Input: part model. Units: mm. Frame: model coordinates. A direction names the side the tool comes from. Coordinates: 2 decimals unless noted, no trailing zeros. Write each loop counter-clockwise with the first axis right and the second up, starting at its lowest first coordinate (ties: lowest second). Pieces come first, ordered by that corner, then holes. Notation, with made-up numbers: M 23.5,23.5 L 37.5,23.5 A22 cw 37.5,32.5 Z; hole C -40,51.25 d1. An arc over 180 degrees is marked long. Write each question's results on one line, items separated by ' | '. Start each with the question number.
1. Set-up query: faces 3 (the flat face through (28, 9.5, 3)), 4 (the flat face through (-8, 20, -2.5)), 5 (the flat face through (-0.899, 32.177, 10.325)). Return all of +Z, -Z, +X, -X, +Y, -Y with unobstructed straight access to the full face (end or side cutting, diameter ignored); none if empty.
2. Ray query, probe 1 along Z at (x, y) = (0.5, 2.8); probe 2 along X at (y, z) = (10, -4); probe 3 along X at (y, z) = (8, -1). Return the intervals inside material, ascending.
3. Section query A-A, the plane x = 0.5. Count the separate pieces of the cut face and the enclosed holes in it, and give its area (3 significant figures).
4. Section query D-D, the plane y = 8.5. Output: boundary loops of the cut face in (x, z), and give its area (3 significant figures).
5. Pull-direction query (X, two-part tool) for faces 1 (the flat face through (12.79, 11.83, -0.26)), 2 (the flat face through (28, 7.5, 3)); classes: +X half, -X half, draft (parallel to the pull), parting line (faces both ways), or undercut.
6. Section query B-B, the plane z = 3.5. Output: boundary loops of the cut face in (x, y), and give its area (3 significant figures).
7. First-contact query: pin 1 (1.5 mm diameter, centred on x = -12.5, y = 33, fed in from +Z); pin 2 (12 mm diameter, centred on x = -17, z = -11.5, fed in from +Y); pin 3 (2.5 mm diameter, centred on x = 24, y = 8, fed in from -Z). Flat tips, straight axial feed; report the tip coordinate or a pass-through.
```python
from build123d import *

# Parameters (mm, degrees)
SKETCH2_W           = 58
SKETCH2_H           = 37
BOSS_EXTRUDE1_DEPTH = 17
BOSS_EXTRUDE2_DEPTH = 58
SKETCH4_R           = 12.5
BOSS_EXTRUDE3_DEPTH = 17
CUT_EXTRUDE1_DEPTH  = 38
SKETCH6_R           = 4.076
CUT_EXTRUDE2_DEPTH  = 23
SKETCH7_R           = 7.5075
SKETCH7_R_2         = 5.15
CUT_EXTRUDE3_DEPTH  = 59
SKETCH8_R           = 1.875
CUT_EXTRUDE4_DEPTH  = 59
SKETCH12_W          = 2
SKETCH12_H          = 2
CUT_EXTRUDE6_DEPTH  = 8
CUT_EXTRUDE7_DEPTH  = 57
SKETCH14_R          = 1.5
CUT_EXTRUDE8_DEPTH  = 35.5


with BuildPart() as part:
    # Sketch2 → Boss-Extrude1 (new body)
    with BuildSketch(Plane(origin=(0, 0, 0), x_dir=(1, 0, 0), z_dir=(0, 1, 0))):
        Rectangle(SKETCH2_W, SKETCH2_H)
    extrude(amount=BOSS_EXTRUDE1_DEPTH)

    # Sketch3 → Boss-Extrude2 (add)
    with BuildSketch(Plane(origin=(29, 0, 0), x_dir=(0, 0, -1), z_dir=(1, 0, 0))):
        with BuildLine():
            Line((-18.5, 23.5), (-18.5, 17))
            Line((-18.5, 17), (2.5, 17))
            Line((2.5, 17), (2.5, 23.5))
            ThreePointArc((2.5, 23.5), (-8, 34), (-18.5, 23.5))
        make_face()
    extrude(amount=-BOSS_EXTRUDE2_DEPTH)

    # Sketch4 → Boss-Extrude3 (add)
    with BuildSketch(Plane(origin=(29, 0, 0), x_dir=(0, 0, -1), z_dir=(1, 0, 0))):
        with Locations((7.043560763, 22)):
            Circle(SKETCH4_R)
    extrude(amount=-BOSS_EXTRUDE3_DEPTH)

    # Sketch5 → Cut-Extrude1 (cut, through all)
    with BuildSketch(Plane(origin=(0, 0, -18.5), x_dir=(-1, 0, 0), z_dir=(0, 0, -1))):
        Polygon((-15.5, 6.5), (-15.5, 10.35), (-10, 13.35), (9, 13.35), (14.5, 10.357), (14.5, 6.5), (9, 3.5), (-10, 3.5), align=None)
    extrude(amount=-CUT_EXTRUDE1_DEPTH, mode=Mode.SUBTRACT)

    # Sketch6 → Cut-Extrude2 (cut)
    with BuildSketch(Plane(origin=(0, 0, -18.5), x_dir=(-1, 0, 0), z_dir=(0, 0, -1))):
        with Locations((-23, 8.5)):
            Circle(SKETCH6_R)
        with Locations((22, 8.5)):
            Circle(SKETCH6_R)
    extrude(amount=-CUT_EXTRUDE2_DEPTH, mode=Mode.SUBTRACT)

    # Sketch7 → Cut-Extrude3 (cut, through all)
    with BuildSketch(Plane(origin=(29, 0, 0), x_dir=(0, 0, -1), z_dir=(1, 0, 0))):
        with Locations((-8, 23.5)):
            Circle(SKETCH7_R)
        with Locations((7.7501439, 23.5)):
            Circle(SKETCH7_R_2)
    extrude(amount=-CUT_EXTRUDE3_DEPTH, mode=Mode.SUBTRACT)

    # Sketch8 → Cut-Extrude4 (cut, through all)
    with BuildSketch(Plane(origin=(29, 0, 0), x_dir=(0, 0, -1), z_dir=(1, 0, 0))):
        with Locations((5.509653427, 31.309982551)):
            Circle(SKETCH8_R)
        with Locations((15.560126451, 25.740490473)):
            Circle(SKETCH8_R)
    extrude(amount=-CUT_EXTRUDE4_DEPTH, mode=Mode.SUBTRACT)

    # Sketch12 → Cut-Extrude6 (cut)
    with BuildSketch(Plane.ZY.offset(29)):
        with Locations((3.5, 8.5)):
            Rectangle(SKETCH12_W, SKETCH12_H)
    cut_extrude6 = extrude(amount=-CUT_EXTRUDE6_DEPTH, mode=Mode.SUBTRACT)

    # Mirror1: Cut-Extrude6 across plane
    add(cut_extrude6.mirror(Plane(origin=(0, 0, 0), x_dir=(0, 0, 1), z_dir=(1, 0, 0))), mode=Mode.SUBTRACT)

    # Sketch13 → Cut-Extrude7 (cut)
    with BuildSketch(Plane.ZY.offset(29)):
        with BuildLine():
            ThreePointArc((8, 31.0075), (8.979925388, 30.943272297), (9.943083981, 30.751688141))
            Line((9.943083981, 30.751688141), (10.717599974, 33.642221176))
            ThreePointArc((10.717599974, 33.642221176), (9.370525018, 33.910171044), (8, 34))
            Line((8, 34), (8, 31.0075))
        make_face()
    extrude(amount=-CUT_EXTRUDE7_DEPTH, mode=Mode.SUBTRACT)

    # Sketch14 → Cut-Extrude8 (cut, through all)
    with BuildSketch(Plane.XZ):
        with Locations((0.5, -11.5)):
            Circle(SKETCH14_R)
    extrude(amount=-CUT_EXTRUDE8_DEPTH, mode=Mode.SUBTRACT)


solid = part.part
```
Answer:
1) face 3: +X | face 4: -Z, -X, +Y | face 5: -X, +Y
2) probe 1: -18.5 to -13, -10 to 18.5 | probe 2: -29 to -25.79, -18.21 to -14.5, 15.5 to 19.21, 26.79 to 29 | probe 3: -29 to -26.05, -17.95 to -14.5, 15.5 to 18.95, 27.05 to 29
3) separate pieces: 4 | enclosed holes: 0 | area: 369 mm^2
4) outline: M -29,-18.5 L -26.08,-18.5 L -26.08,2.5 L -29,2.5 Z; M -29,4.5 L -17.92,4.5 L -17.92,-18.5 L -14.5,-18.5 L -14.5,18.5 L -29,18.5 Z; M 15.5,-18.5 L 18.92,-18.5 L 18.92,4.5 L 29,4.5 L 29,18.5 L 15.5,18.5 Z; M 27.08,-18.5 L 29,-18.5 L 29,2.5 L 27.08,2.5 Z | area: 651 mm^2
5) face 1: undercut | face 2: draft
6) outline: M -29,0 L 29,0 L 29,7.5 L 26.95,7.5 A4.08 cw long 26.95,9.5 L 29,9.5 L 29,17.49 L -29,17.49 L -29,9.5 L -25.95,9.5 A4.08 cw long -25.95,7.5 L -29,7.5 Z; M -29,29.51 L 29,29.51 L 29,32.99 L -29,32.99 Z; hole M -14.5,6.5 L -9,3.5 L 10,3.5 L 15.5,6.5 L 15.5,10.35 L 10,13.35 L -9,13.35 L -14.5,10.36 Z | area: 839 mm^2
7) pin 1: z = 13.8 | pin 2: y = 17 | pin 3: z = 4.5
